from build123d import *

# Parameters (mm, degrees)
F0_R     = 5
F1_DEPTH = 30
F2_R     = 10.25
F3_DEPTH = 55
F4_R     = 6.75
F5_DEPTH = 45
F6_SIZE2 = 0.2679491924
F6_SIZE  = 1
F7_R     = 2
F8_DEPTH = 10


with BuildPart() as f1:
    # F0 (on Top) → F1 (new body)
    with BuildSketch(Plane.XY):
        Circle(F0_R)
    extrude(amount=F1_DEPTH)

    # F2 (on face) → F3 (join)
    with BuildSketch(Plane.XY.offset(30)):
        Circle(F2_R)
    extrude(amount=F3_DEPTH)

    # F4 (on face) → F5 (cut)
    with BuildSketch(Plane.XY.offset(85)):
        Circle(F4_R)
    extrude(amount=-F5_DEPTH, mode=Mode.SUBTRACT)

    # F6
    f6_edges = [f1.edges().sort_by_distance(p)[0] for p in [
        (-10.25, 0, 85),
    ]]
    f6_side = f1.faces().sort_by_distance((-9.960086, 0, 85))[0]
    chamfer(f6_edges, length=F6_SIZE, length2=F6_SIZE2, reference=f6_side)

    # F7 (on Front) → F8 (cut, symmetric)
    with BuildSketch(Plane.XZ):
        with Locations((0, 10)):
            Circle(F7_R)
    extrude(amount=F8_DEPTH, both=True, mode=Mode.SUBTRACT)


solid = f1.part
For this review, take the finished solid that the model builds, in its own axes (mm). A direction names the side the tool comes from. Round coordinates to 2 decimals unless told otherwise and drop trailing zeros. Order: outer loops, then holes, each group sorted by start corner. A loop starts at its lowest first (then second) coordinate and runs counter-clockwise, first axis right, second up. Notation, with made-up numbers: M -13.5,-36.5 L 13.5,-36.5 A30 ccw 13.5,-0.5 Z; hole C 30,-35.75 d10. An arc over 180 degrees is marked long. Use a Markdown table: item, result. Add a question column.
Item 1: Add section D-D, the plane z = 21. Give the boundary of the cut face in (x, y).
Item 2: Add section A-A, the plane x = 0. Give the boundary of the cut face in (y, z).
Item 3: Add section C-C, the plane z = 75. Give the boundary of the cut face in (x, y).
Item 4: Tool access review of faces 1 (the cylindrical face through (-1.46, -6.59, 62.82)), 2 (the flat face through (0, 0, 0)), 3 (the flat face through (2, 5, 30)): name each direction out of +Z, -Z, +X, -X, +Y, -Y from which nothing blocks a thin tool from reaching the whole face with its end or side.
Item 5: To check wall thickness, follow line 1 along Z through (x, y) = (0, 1.25); line 2 along Y through (x, z) = (0, 64); line 3 along X through (y, z) = (0.25, 15). State the ranges of each line that lie inside material, in increasing order.
Item 6: Insertion check: pin 1 (8 mm diameter, centred on y = -7.5, z = 30.5, fed in from +X); pin 2 (1.5 mm diameter, centred on x = 0.5, y = -0.5, fed in from +Z); pin 3 (2.5 mm diameter, centred on x = 0, z = 10, fed in from +Y); pin 4 (10 mm diameter, centred on y = 3.5, z = 38.5, fed in from +X). Each pin has a flat end and moves straight along its axis. Give the tip position at first contact, or say it passes through.
Item 7: Mouldability with a two-part tool opening along X and no side actions: class faces 4 (the flat face through (1, -7, 85)), 5 (the cylindrical face through (0, 0, 12)), 6 (the cylindrical face through (2.307, -4.436, 14.79)), 7 (the flat face through (0, 0, 40)) as released by +X, released by -X, zero draft, split by the parting line, or undercut.
Item 8: Add section B-B, the plane y = 0. Give the boundary of the cut face in (x, z), then the cut area to 3 significant figures.
Geometry results:
| question | item | result |
|---|---|---|
| 1 | outline | C 0,0 d10 |
| 2 | outline | M -10.25,30 L -5,30 L -5,12 L 5,12 L 5,30 L 10.25,30 L 10.25,84.73 L 9.25,85 L 6.75,85 L 6.75,40 L -6.75,40 L -6.75,85 L -9.25,85 L -10.25,84.73 Z; M -5,0 L 5,0 L 5,8 L -5,8 Z |
| 3 | outline | C 0,0 d20.5; hole C 0,0 d13.5 |
| 4 | face 1 | +Z |
| 4 | face 2 | -Z, +X, -X, +Y, -Y |
| 4 | face 3 | -Z |
| 5 | line 1 | z = 0 to 8, 12 to 40 |
| 5 | line 2 | y = -10.25 to -6.75, 6.75 to 10.25 |
| 5 | line 3 | x = -4.99 to 4.99 |
| 6 | pin 1 | stops at x = 9.63 |
| 6 | pin 2 | stops at z = 40 |
| 6 | pin 3 | passes through |
| 6 | pin 4 | stops at x = 10.25 |
| 7 | face 4 | zero draft |
| 7 | face 5 | undercut |
| 7 | face 6 | split by the parting line |
| 7 | face 7 | undercut |
| 8 | outline | M -10.25,30 L -5,30 L -5,0 L 5,0 L 5,30 L 10.25,30 L 10.25,84.73 L 9.25,85 L 6.75,85 L 6.75,40 L -6.75,40 L -6.75,85 L -9.25,85 L -10.25,84.73 Z; hole C 0,10 d4 |
| 8 | area | 807 mm² |
